The listing builds one solid part. Answer for the finished solid, in the listing's coordinates (mm). A direction names the side the tool comes from. Round coordinates to 2 decimals unless told otherwise and drop trailing zeros. Loops run counter-clockwise (first coordinate to the right, second up) from the corner with the lowest first, then second, coordinate; pieces in that order, holes last. Notation, with made-up numbers: (18, 51) -> (39, 51) arc R9 cw to (39, 62) -> close; hole circle Ø10 at (15.5, -40). An arc over 180 degrees is marked (long way). Use a Markdown table: item, result. Add a question column.
Q1. Consider line 1 (Z direction, x = 11.5, y = -7.5); line 2 (X direction, y = 30.5, z = 51.5). Determine where each line is inside the solid, lowest interval first.
Q2. Section B-B on x = 31 is taken. Give the vertices of the cut face in (y, z).
Q3. Given pin 1 Ø10 at (y, z) = (0, 8) entering from +X, flat-ended and moving along its own axis, determine where the tip first touches the part or whether it passes through.
Q4. Which of the six approach directions +Z, -Z, +X, -X, +Y, -Y give full straight-line access (tool end or side, diameter ignored) to faces 5 (the flat face through (35, -30, 29)), 6 (the flat face through (-40, -27.5, 29)), 7 (the flat face through (-1, 0, 57))?
Q5. For a pull along Y with two mould halves and no side action, classify faces 1 (the flat face through (0, -32.5, 1)), 2 (the flat face through (40, -27.5, 29)), 3 (the flat face through (-1, 0, 59)), 4 (the flat face through (0, 32.5, 1)) as released by +Y, released by -Y, zero draft, split by the parting line, or undercut.
Q6. Section A-A on z = 41 is taken. Give the vertices of the cut face in (x, y), then the cut area to 3 significant figures.
Q7. Section C-C on y = -13.5 is taken. Give the vertices of the cut face in (x, z), then the cut area to 3 significant figures.
from build123d import *

# Parameters (mm, degrees)
SKETCH1_W                                  = 90
SKETCH1_H                                  = 65
BOSS_EXTRUDE1_DEPTH                        = 2
SKETCH2_W                                  = 10
SKETCH2_H                                  = 5
BOSS_EXTRUDE2_DEPTH                        = 55
MIRROR1_AT_THE_SECOND_PLANE_COPY_1_SKETC_W = 10
MIRROR1_AT_THE_SECOND_PLANE_COPY_1_SKETC_H = 5
MIRROR1_AT_THE_SECOND_PLANE_COPY_1_DEPTH   = 55
SKETCH3_W                                  = 90
SKETCH3_H                                  = 65
BOSS_EXTRUDE3_DEPTH                        = 2


with BuildPart() as part:
    # Sketch1 → Boss-Extrude1 (new body)
    with BuildSketch(Plane.XY):
        Rectangle(SKETCH1_W, SKETCH1_H)
    extrude(amount=BOSS_EXTRUDE1_DEPTH)

    # Sketch2 → Boss-Extrude2 (add)
    with BuildSketch(Plane.XY.offset(2)):
        with Locations((-40, 30)):
            Rectangle(SKETCH2_W, SKETCH2_H)
    boss_extrude2 = extrude(amount=BOSS_EXTRUDE2_DEPTH)

    # Mirror1: Boss-Extrude2 across plane
    add(boss_extrude2.mirror(Plane(origin=(0, 0, 0), x_dir=(0, 0, 1), z_dir=(1, 0, 0))))

    # Mirror1 at the second plane: Boss-Extrude2 across plane
    add(boss_extrude2.mirror(Plane.ZX))

    # Mirror1 at the second plane copy 1 sketc → Mirror1 at the second plane copy 1 (add)
    with BuildSketch(Plane(origin=(0, 0, 2), x_dir=(-1, 0, 0), z_dir=(0, 0, 1))):
        with Locations((-40, 30)):
            Rectangle(MIRROR1_AT_THE_SECOND_PLANE_COPY_1_SKETC_W, MIRROR1_AT_THE_SECOND_PLANE_COPY_1_SKETC_H)
    extrude(amount=MIRROR1_AT_THE_SECOND_PLANE_COPY_1_DEPTH)

    # Sketch3 → Boss-Extrude3 (add)
    with BuildSketch(Plane.XY.offset(57)):
        Rectangle(SKETCH3_W, SKETCH3_H)
    extrude(amount=BOSS_EXTRUDE3_DEPTH)


solid = part.part
Checked values:
| question | item | result |
|---|---|---|
| 1 | line 1 | z = 0 to 2, 57 to 59 |
| 1 | line 2 | x = -45 to -35, 35 to 45 |
| 2 | outline | (-32.5, 0) -> (32.5, 0) -> (32.5, 2) -> (-32.5, 2) -> close; (-32.5, 57) -> (32.5, 57) -> (32.5, 59) -> (-32.5, 59) -> close |
| 3 | pin 1 | passes through |
| 4 | face 5 | +Y, -Y |
| 4 | face 6 | +X, -X |
| 4 | face 7 | none |
| 5 | face 1 | released by -Y |
| 5 | face 2 | undercut |
| 5 | face 3 | zero draft |
| 5 | face 4 | released by +Y |
| 6 | outline | (-45, -32.5) -> (-35, -32.5) -> (-35, -27.5) -> (-45, -27.5) -> close; (-45, 27.5) -> (-35, 27.5) -> (-35, 32.5) -> (-45, 32.5) -> close; (35, -32.5) -> (45, -32.5) -> (45, -27.5) -> (35, -27.5) -> close; (35, 27.5) -> (45, 27.5) -> (45, 32.5) -> (35, 32.5) -> close |
| 6 | area | 200 mm2 |
| 7 | outline | (-45, 0) -> (45, 0) -> (45, 2) -> (-45, 2) -> close; (-45, 57) -> (45, 57) -> (45, 59) -> (-45, 59) -> close |
| 7 | area | 360 mm2 |
